Design review of the part built by this model. Coordinates are the model's own, in mm. A direction names the side the tool comes from. Coordinates: 2 decimals unless noted, no trailing zeros. Loops run counter-clockwise (first coordinate to the right, second up) from the corner with the lowest first, then second, coordinate; pieces in that order, holes last. Notation, with made-up numbers: M -32,51 L 23,51 A19 ccw 23,82 Z; hole C -23.5,25.5 d5. An arc over 180 degrees is marked long. One line per item, written item: value.
```python
from build123d import *

# Parameters (mm, degrees)
SKETCH_W     = 36.74
SKETCH_H     = 16.2
SKETCH_R     = 0.9
PAD_DEPTH    = 0.8
SKETCH001_W  = 13.34
SKETCH001_H  = 16.2
SKETCH001_R  = 0.9
PAD001_DEPTH = 1
SKETCH002_W  = 22.987506
SKETCH002_H  = 9.9264
POCKET_DEPTH = 0.801


with BuildPart() as part:
    # Sketch → Pad (new body)
    with BuildSketch(Plane.XY):
        with Locations((-15.4, 34.77)):
            Rectangle(SKETCH_W, SKETCH_H)
        with Locations((1.83, 39.2)):
            Circle(SKETCH_R, mode=Mode.SUBTRACT)
        with Locations((1.83, 30)):
            Circle(SKETCH_R, mode=Mode.SUBTRACT)
        with Locations((-31.67, 39.2)):
            Circle(SKETCH_R, mode=Mode.SUBTRACT)
        with Locations((-31.67, 30)):
            Circle(SKETCH_R, mode=Mode.SUBTRACT)
    extrude(amount=PAD_DEPTH)

    # Sketch001 (on Face10 of Pad) → Pad001 (join)
    with BuildSketch(Plane.XY.offset(0.8)):
        with Locations((-3.7, 34.77)):
            Rectangle(SKETCH001_W, SKETCH001_H)
        with Locations((1.83, 39.2)):
            Circle(SKETCH001_R, mode=Mode.SUBTRACT)
        with Locations((1.83, 30)):
            Circle(SKETCH001_R, mode=Mode.SUBTRACT)
    extrude(amount=PAD001_DEPTH)

    # Sketch002 (on Face3 of Pad001) → Pocket (cut, through all)
    with BuildSketch(Plane.XY.offset(0.8)):
        with Locations((-23.321447, 34.5539)):
            Rectangle(SKETCH002_W, SKETCH002_H)
    extrude(amount=-POCKET_DEPTH, mode=Mode.SUBTRACT)


solid = part.part
```
(1) We need section A-A on y = 30. State the section outline as (x, z) points.
Reply:
outline: M -11.83,0 L 0.93,0 L 0.93,1.8 L -10.37,1.8 L -10.37,0.8 L -11.83,0.8 Z; M 2.73,0 L 2.97,0 L 2.97,1.8 L 2.73,1.8 Z
(2) Insertion check: pin 1 (3 mm diameter, centred on x = -24, y = 31.5, fed in from +Z); pin 2 (2 mm diameter, centred on x = 1.83, y = 39.2, fed in from +Z). Each pin has a flat end and moves straight along its axis. Give the tip position at first contact, or say it passes through.
Reply:
pin 1: passes through
pin 2: stops at z = 1.8
(3) Mouldability with a two-part tool opening along Y and no side actions: class faces 1 (the cylindrical face through (2.31, 39.96, 0.89)), 2 (the flat face through (2.97, 35, 1)), 3 (the flat face through (-11.6, 26.67, 0.5)) as released by +Y, released by -Y, zero draft, split by the parting line, or undercut.
Reply:
face 1: undercut
face 2: zero draft
face 3: released by -Y
(4) Tool access review of faces 4 (the cylindrical face through (1.12, 29.45, 0.89)), 5 (the flat face through (-22, 40, 0.8)): name each direction out of +Z, -Z, +X, -X, +Y, -Y from which nothing blocks a thin tool from reaching the whole face with its end or side.
Reply:
face 4: +Z, -Z
face 5: +Z, -X, +Y, -Y
(5) To check wall thickness, follow line 1 along Y through (x, z) = (1.83, 0.5); line 2 along Y through (x, z) = (-24.5, 0.1); line 3 along X through (y, z) = (39.2, 1.2). State the ranges of each line that lie inside material, in increasing order. Write a range as [from, to].
Reply:
line 1: y = [26.67, 29.1], [30.9, 38.3], [40.1, 42.87]
line 2: y = [26.67, 29.59], [39.52, 42.87]
line 3: x = [-10.37, 0.93], [2.73, 2.97]
(6) We need section B-B on z = 0.4. State the section outline as (x, y) points.
Reply:
outline: M -33.77,26.67 L 2.97,26.67 L 2.97,42.87 L -33.77,42.87 L -33.77,39.52 L -32.51,39.52 A0.9 cw -30.83,39.52 L -11.83,39.52 L -11.83,29.59 L -30.87,29.59 A0.9 cw -32.47,29.59 L -33.77,29.59 Z; hole C 1.83,30 d1.8; hole C 1.83,39.2 d1.8
(7) We need section D-D on x = -14. State the section outline as (y, z) points.
Reply:
outline: M 26.67,0 L 29.59,0 L 29.59,0.8 L 26.67,0.8 Z; M 39.52,0 L 42.87,0 L 42.87,0.8 L 39.52,0.8 Z
(8) We need section C-C on x = 1.83. State the section outline as (y, z) points, then the cut area to 3 significant figures.
Reply:
outline: M 26.67,0 L 29.1,0 L 29.1,1.8 L 26.67,1.8 Z; M 30.9,0 L 38.3,0 L 38.3,1.8 L 30.9,1.8 Z; M 40.1,0 L 42.87,0 L 42.87,1.8 L 40.1,1.8 Z
area: 22.7 mm2
